Design review of the part built by this model. Coordinates are the model's own, in mm. A direction names the side the tool comes from. Round coordinates to 2 decimals unless told otherwise and drop trailing zeros. Loops run counter-clockwise (first coordinate to the right, second up) from the corner with the lowest first, then second, coordinate; pieces in that order, holes last. Notation, with made-up numbers: (60.5, 41) - (95.5, 41) arc R38 cw to (95.5, 80) - close; hole circle Ø6 at (-16.75, -0.5). An arc over 180 degrees is marked (long way). Answer as CSV lines item,"result". Start each with the question number.
(1) Consider section B-B (z = 0). Give the boundary of the cut face in (x, y).
(2) Consider section C-C (y = -4.75). Give the boundary of the cut face in (x, z), and give its area (3 significant figures).
(3) Consider section A-A (x = 0). Give the boundary of the cut face in (y, z), and give its area (3 significant figures).
(4) For P1, Ø4, axis at y = -0.5, z = 7, coming from the +X side; P2, Ø2, axis at y = -4.5, z = -6.5, coming from the -X side; P3, Ø5, axis at y = -4.5, z = 5, coming from the +X side, all flat-tipped, find the tip position at first contact; note any pin that passes through.
(5) For faces 1 (the flat face through (2, -8.5, -9)), 2 (the cylindrical face through (-2.38, 11.95, -10.74)), list the 3-axis set-ups (+Z, -Z, +X, -X, +Y, -Y) from which the entire face can be reached by the end or side of a thin tool; tool diameter is ignored.
(6) Consider section D-D (x = -5.5). Give the boundary of the cut face in (y, z), and give its area (3 significant figures).
(7) Mouldability with a two-part tool opening along Y and no side actions: class faces 3 (the flat face through (2, 8.5, -9)), 4 (the cylindrical face through (-2.38, -9.01, -10.74)), 5 (the flat face through (2, -9.5, -5)) as released by +Y, released by -Y, zero draft, split by the parting line, or undercut.
(8) Wall thickness on L1, parallel to Y at x = 6.75, z = 6; L2, parallel to Z at x = -3.75, y = 10.25; L3, parallel to X at y = -7, z = -2.25: over which ranges is each line inside the solid? List them lowest first.
from build123d import *

# Parameters (mm, degrees)
F0_R     = 9
F1_DEPTH = 9.5
F2_R     = 11
F3_DEPTH = 1
F5_DEPTH = 6
F6_R     = 5
F7_DEPTH = 25


with BuildPart() as f1:
    # F0 (on Front) → F1 (new body)
    with BuildSketch(Plane.XZ):
        Circle(F0_R)
    extrude(amount=F1_DEPTH)

    # F2 (on face) → F3 (join)
    with BuildSketch(Plane.XZ.offset(9.5)):
        Circle(F2_R)
    extrude(amount=-F3_DEPTH)

    # F4: F1 across plane


with BuildPart() as f1_1:
    add(f1.part)
    add(f1.part.mirror(Plane.XZ))

    # F5 (add): a face of the model
    f5_faces = [f1_1.faces().sort_by_distance(p)[0] for p in [
        (0, 9.5, 0),
    ]]
    extrude(f5_faces, amount=F5_DEPTH)

    # F6 (on face) → F7 (cut)
    with BuildSketch(Plane.XZ.offset(9.5)):
        Circle(F6_R)
    extrude(amount=-F7_DEPTH, mode=Mode.SUBTRACT)


solid = f1_1.part
Determined:
1,outline,"(-11, -9.5) - (-5, -9.5) - (-5, 15.5) - (-11, 15.5) - (-11, 8.5) - (-9, 8.5) - (-9, -8.5) - (-11, -8.5) - close; (5, -9.5) - (11, -9.5) - (11, -8.5) - (9, -8.5) - (9, 8.5) - (11, 8.5) - (11, 15.5) - (5, 15.5) - close"
2,outline,"circle Ø18 at (0, 0); hole circle Ø10 at (0, 0)"
2,area,"176 mm^2"
3,outline,"(-9.5, -11) - (-8.5, -11) - (-8.5, -9) - (8.5, -9) - (8.5, -11) - (15.5, -11) - (15.5, -5) - (-9.5, -5) - close; (-9.5, 5) - (15.5, 5) - (15.5, 11) - (8.5, 11) - (8.5, 9) - (-8.5, 9) - (-8.5, 11) - (-9.5, 11) - close"
3,area,"232 mm^2"
4,P1,"stops at x = 7.48"
4,P2,"stops at x = -7.12"
4,P3,"stops at x = 8.65"
5,face 1,"none"
5,face 2,"+Y, -Y"
6,outline,"(-9.5, -9.53) - (-8.5, -9.53) - (-8.5, -7.12) - (8.5, -7.12) - (8.5, -9.53) - (15.5, -9.53) - (15.5, 9.53) - (8.5, 9.53) - (8.5, 7.12) - (-8.5, 7.12) - (-8.5, 9.53) - (-9.5, 9.53) - close"
6,area,"395 mm^2"
7,face 3,"undercut"
7,face 4,"zero draft"
7,face 5,"released by -Y"
8,L1,"y = -9.5 to -8.5, 8.5 to 15.5"
8,L2,"z = -10.34 to -3.31, 3.31 to 10.34"
8,L3,"x = -8.71 to -4.47, 4.47 to 8.71"
